Here's the drawing with two shaded views (mm, measured from the low corner). I have some questions. A direction names the side the tool comes from. Round coordinates to 2 decimals unless told otherwise and drop trailing zeros. Order: outer loops, then holes, each group sorted by start corner. A loop starts at its lowest first (then second) coordinate and runs counter-clockwise, first axis right, second up. Notation, with made-up numbers: (37.5, 1.25) -> (83.5, 1.25) arc R13 ccw to (83.5, 13.25) -> close; hole circle Ø11 at (-35, 14). An arc over 180 degrees is marked (long way). Answer in a Markdown table with one row per item.
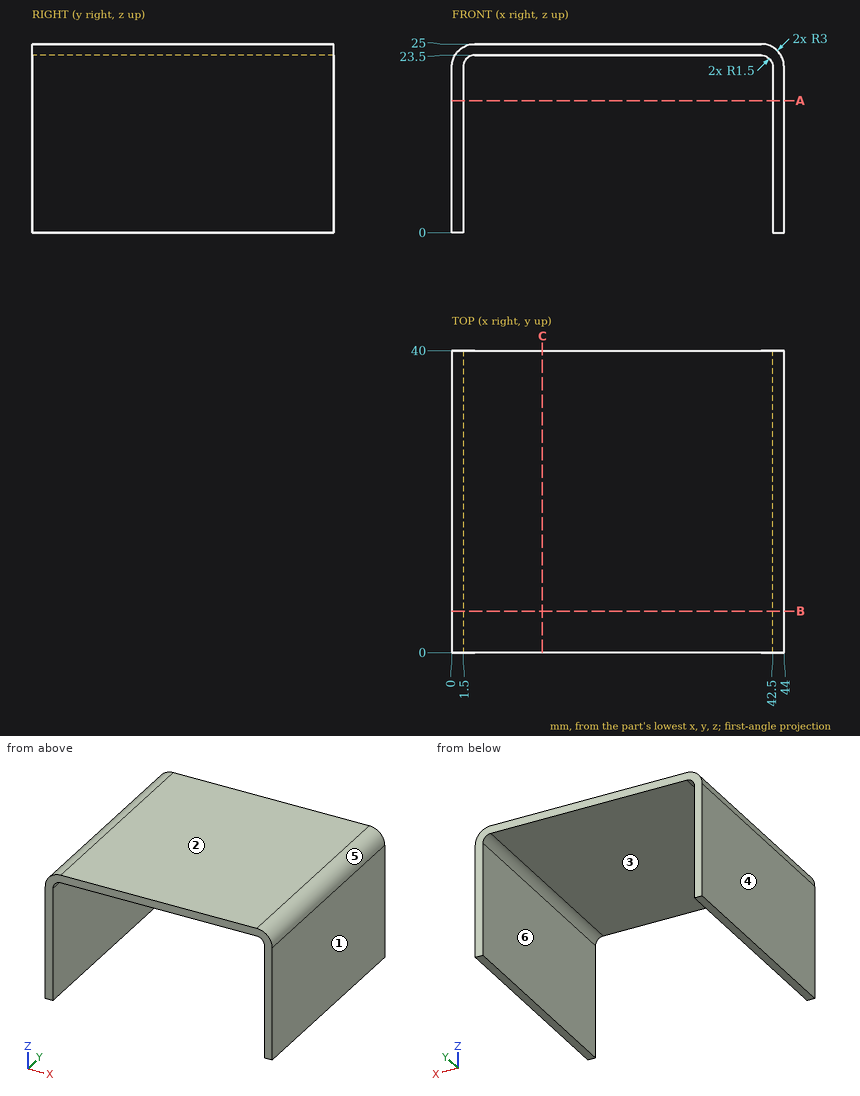
1. Suppose I cut it at A-A on z = 17.5. Write out the boundary of the cut face in (x, y).
Numbers:
| item | result |
|---|---|
| outline | (0, 0) -> (1.5, 0) -> (1.5, 40) -> (0, 40) -> close; (42.5, 0) -> (44, 0) -> (44, 40) -> (42.5, 40) -> close |
2. We'd pull the mould along X, two halves only. Please class the marked faces 1, 2, 3 and 4: released by +X, released by -X, zero draft, split by the parting line, or undercut.
Numbers:
| item | result |
|---|---|
| face 1 | released by +X |
| face 2 | zero draft |
| face 3 | undercut |
| face 4 | released by -X |
3. For the marked faces 5 and 6, which set-ups out of +Z, -Z, +X, -X, +Y, -Y let a thin tool reach every point of the face, with its end or its side?
Numbers:
| item | result |
|---|---|
| face 5 | +Z, +X, +Y, -Y |
| face 6 | -Z, +Y, -Y |
4. Suppose I cut it at C-C on x = 12. Write out the boundary of the cut face in (y, z).
Numbers:
| item | result |
|---|---|
| outline | (0, 23.5) -> (40, 23.5) -> (40, 25) -> (0, 25) -> close |
5. For pin 1 Ø3 at (x, y) = (16.5, 5) entering from -Z, with a flat end and sliding along its axis, tell me the tip position at first contact or that it passes through.
Numbers:
| item | result |
|---|---|
| pin 1 | stops at z = 23.5 |
6. Please list where these lines run through material, in increasing order: line 1 along X through (y, z) = (23, 13.25); line 2 along Z through (x, y) = (11, 19.5); line 3 along X through (y, z) = (37.5, 24).
Numbers:
| item | result |
|---|---|
| line 1 | x = 0 to 1.5, 42.5 to 44 |
| line 2 | z = 23.5 to 25 |
| line 3 | x = 0.76 to 43.24 |
7. Suppose I cut it at B-B on y = 5.5. Write out the boundary of the cut face in (x, z).
Numbers:
| item | result |
|---|---|
| outline | (0, 0) -> (1.5, 0) -> (1.5, 22) arc R1.5 cw to (3, 23.5) -> (41, 23.5) arc R1.5 cw to (42.5, 22) -> (42.5, 0) -> (44, 0) -> (44, 22) arc R3 ccw to (41, 25) -> (3, 25) arc R3 ccw to (0, 22) -> close |
